Check sheet for the drawn part. Datum: minimum x, y, z corner. Units: mm. Give positions to 0.01 mm unless a question says otherwise; leave off trailing zeros. Loops run counter-clockwise (first coordinate to the right, second up) from the corner with the lowest first, then second, coordinate; pieces in that order, holes last. Notation, with made-up numbers: (26, 60) - (45, 60) arc R13 cw to (45, 83) - close; hole circle Ø10 at (27, 72.5). An arc over 180 degrees is marked (long way). Use one line per item in the form item = value.
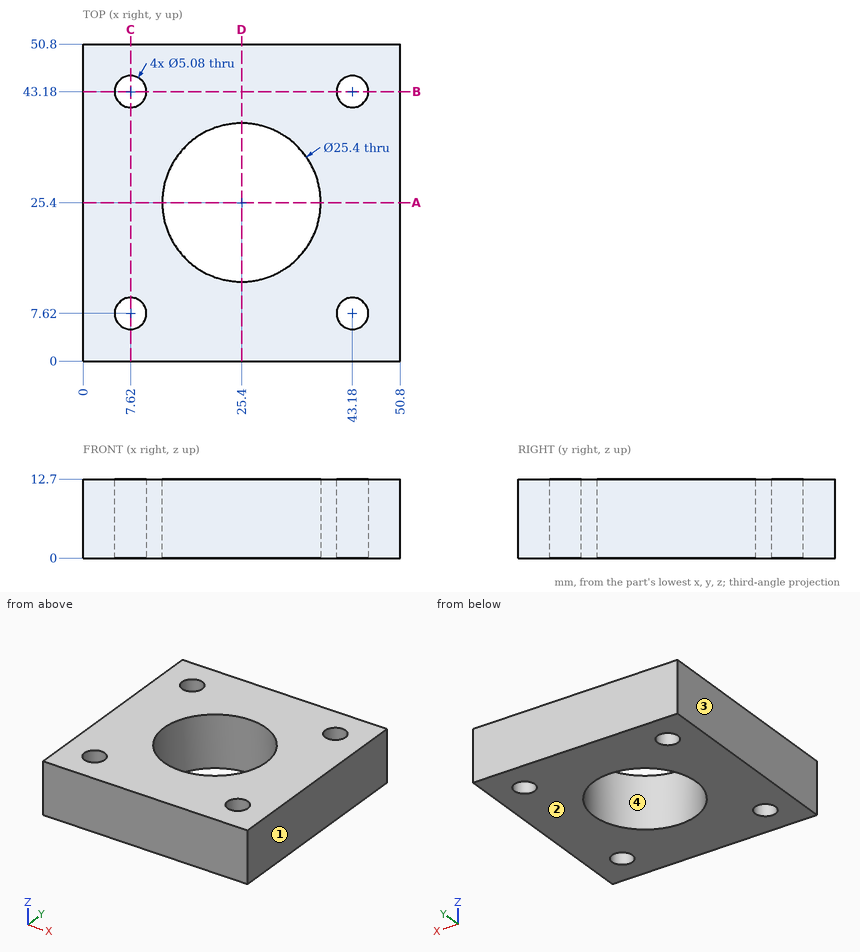
1. Draft check along X on the marked faces 1, 2, 3 and 4. Enter one of: released by +X, released by -X, zero draft, split by the parting line, or undercut.
Result set:
face_1 = released by +X
face_2 = zero draft
face_3 = released by -X
face_4 = undercut
2. Section check B-B, the plane y = 43.18. Record the cut outline in (x, z).
Result set:
outline = (0, 0) - (5.08, 0) - (5.08, 12.7) - (0, 12.7) - close; (10.16, 0) - (40.64, 0) - (40.64, 12.7) - (10.16, 12.7) - close; (45.72, 0) - (50.8, 0) - (50.8, 12.7) - (45.72, 12.7) - close
3. Section check A-A, the plane y = 25.4. Record the cut outline in (x, z), then the cut area to 3 significant figures.
Result set:
outline = (0, 0) - (12.7, 0) - (12.7, 12.7) - (0, 12.7) - close; (38.1, 0) - (50.8, 0) - (50.8, 12.7) - (38.1, 12.7) - close
area = 323 mm²
4. Scan lines: probe 1 along Y at (x, z) = (25.4, 8.5); probe 2 along Y at (x, z) = (7.62, 5); probe 3 along X at (y, z) = (43, 5.5). Record each from-to range of solid material in increasing order.
Result set:
probe_1 = 0 to 12.7, 38.1 to 50.8
probe_2 = 0 to 5.08, 10.16 to 40.64, 45.72 to 50.8
probe_3 = 0 to 5.09, 10.15 to 40.65, 45.71 to 50.8
5. Depth check by flat-ended pin: pin 1 Ø8 at (x, y) = (43.18, 7.62) entering from -Z; pin 2 Ø4.5 at (x, y) = (43.18, 43.18) entering from -Z. Enter the tip coordinate at first touch or a pass-through.
Result set:
pin_1 = 0
pin_2 = through
